```python
from build123d import *

# Parameters (mm, degrees)
SKETCH1_W               = 265
SKETCH1_H               = 340
BOSS_EXTRUDE1_DEPTH     = 50
SKETCH2_R               = 7.5
BOSS_EXTRUDE2_DEPTH     = 80
SKETCH7_R               = 7.5
BOSS_EXTRUDE3_DEPTH     = 80
SKETCH8_R               = 7.5
CUT_EXTRUDE1_DEPTH      = 410
SKETCH9_R               = 7.5
CUT_EXTRUDE2_DEPTH      = 410
CUT_EXTRUDE4_DEPTH      = 463.803826299
CUT_EXTRUDE4_DEPTH_BACK = 463.803826299


with BuildPart() as part:
    # Sketch1 → Boss-Extrude1 (new body)
    with BuildSketch(Plane.XY):
        Polygon((-7.287721529, 248.848476773), (17.712278471, 248.848476773), (17.712278471, -351.151523227), (-7.287721529, -351.151523227), (-7.287721529, -271.151523227), (-272.287721529, -271.151523227), (-272.287721529, -351.151523227), (-297.287721529, -351.151523227), (-297.287721529, 248.848476773), (-272.287721529, 248.848476773), (-272.287721529, 168.848476773), (-7.287721529, 168.848476773), align=None)
        with Locations((-139.787721529, -51.151523227)):
            Rectangle(SKETCH1_W, SKETCH1_H, mode=Mode.SUBTRACT)
    extrude(amount=BOSS_EXTRUDE1_DEPTH)

    # Sketch2 → Boss-Extrude2 (add)
    with BuildSketch(Plane(origin=(17.712278471, 0, 0), x_dir=(0, 0, -1), z_dir=(1, 0, 0))):
        with Locations((-26.558504248, -51.151523227)):
            Circle(SKETCH2_R)
    extrude(amount=-BOSS_EXTRUDE2_DEPTH)

    # Sketch7 → Boss-Extrude3 (add)
    with BuildSketch(Plane.ZY.offset(297.287721529)):
        with Locations((25, -51.151523227)):
            Circle(SKETCH7_R)
    extrude(amount=-BOSS_EXTRUDE3_DEPTH)

    # Sketch8 → Cut-Extrude1 (cut)
    with BuildSketch(Plane.ZY.offset(297.287721529)):
        with Locations((25, -331.151523227)):
            Circle(SKETCH8_R)
    extrude(amount=-CUT_EXTRUDE1_DEPTH, mode=Mode.SUBTRACT)

    # Sketch9 → Cut-Extrude2 (cut)
    with BuildSketch(Plane.ZY.offset(297.287721529)):
        with Locations((25, 228.848476773)):
            Circle(SKETCH9_R)
    extrude(amount=-CUT_EXTRUDE2_DEPTH, mode=Mode.SUBTRACT)

    # Sketch11 → Cut-Extrude4 (cut, two sides: drawn at the far end of the back side and taken through both)
    with BuildSketch(Plane(origin=(0, 0, 0), x_dir=(0, 0, -1), z_dir=(1, 0, 0)).offset(-CUT_EXTRUDE4_DEPTH_BACK)):
        Polygon((-50, -351.151523227), (-28, -351.151523227), (-50, -300.151523227), align=None)
    extrude(amount=CUT_EXTRUDE4_DEPTH + CUT_EXTRUDE4_DEPTH_BACK, mode=Mode.SUBTRACT)


solid = part.part
```
Design review of the part built by this model. Coordinates are the model's own, in mm. A direction names the side the tool comes from. Coordinates: 2 decimals unless noted, no trailing zeros. Order: outer loops, then holes, each group sorted by start corner. A loop starts at its lowest first (then second) coordinate and runs counter-clockwise, first axis right, second up. Notation, with made-up numbers: M 75.25,68.25 L 100.25,68.25 A28 ccw 100.25,101.25 Z; hole C -15,33.25 d6. An arc over 180 degrees is marked long. Answer as a JSON object with one key per item and string values. Group by question number.
1) Mouldability with a two-part tool opening along X and no side actions: class faces 1 (the flat face through (-297.288, -47, 25)), 2 (the flat face through (-278, -47, 0)), 3 (the flat face through (-142, -221.152, 25)) as pulls with the +X half, pulls with the -X half, needs draft (parallel to the pull), parting line crosses it, or undercut.
2) Add section C-C, the plane z = 11. Write out the cut boundary in (x, y).
3) Add section A-A, the plane y = 0.5. Write out the cut boundary in (x, z).
4) Add section D-D, the plane z = 39.5. Write out the cut boundary in (x, y).
5) For pin 1 (1.5 mm diameter, centred on x = -114.5, z = 7, fed in from -Y); pin 2 (2 mm diameter, centred on x = -27, z = 34, fed in from +Y); pin 3 (25 mm diameter, centred on y = -329.5, z = 18.5, fed in from -X), all flat-tipped, find the tip position at first contact; note any pin that passes through.
6) Add section B-B, the plane x = -205. Write out the cut boundary in (y, z), then the cut area to 3 significant figures.
7) Tool access review of faces 4 (the flat face through (-62.288, -51, 27)), 5 (the flat face through (-7.288, -303, 19)), 6 (the flat face through (-272.288, 209, 25)), 7 (the cylindrical face through (-245.173, -46.083, 19.472)): name each direction out of +Z, -Z, +X, -X, +Y, -Y from which nothing blocks a thin tool from reaching the whole face with its end or side.
8) Wall thickness on L1, parallel to Y at x = -26, z = 27; L2, parallel to Y at x = 12.25, z = 25; L3, parallel to X at y = -125.5, z = 38: over which ranges is each line inside the solid? List them lowest first.
Computed values:
{
 "1": {"face 1": "pulls with the -X half", "face 2": "needs draft", "face 3": "undercut"},
 "2": {"outline": "M -297.29,-351.15 L -272.29,-351.15 L -272.29,-271.15 L -7.29,-271.15 L -7.29,-351.15 L 17.71,-351.15 L 17.71,248.85 L -7.29,248.85 L -7.29,168.85 L -272.29,168.85 L -272.29,248.85 L -297.29,248.85 Z; hole M -272.29,-221.15 L -7.29,-221.15 L -7.29,118.85 L -272.29,118.85 Z"},
 "3": {"outline": "M -297.29,0 L -272.29,0 L -272.29,50 L -297.29,50 Z; M -7.29,0 L 17.71,0 L 17.71,50 L -7.29,50 Z"},
 "4": {"outline": "M -297.29,-324.49 L -272.29,-324.49 L -272.29,-271.15 L -7.29,-271.15 L -7.29,-324.49 L 17.71,-324.49 L 17.71,248.85 L -7.29,248.85 L -7.29,168.85 L -272.29,168.85 L -272.29,248.85 L -297.29,248.85 Z; hole M -272.29,-221.15 L -7.29,-221.15 L -7.29,118.85 L -272.29,118.85 Z"},
 "5": {"pin 1": "stops at y = -271.15", "pin 2": "stops at y = 168.85", "pin 3": "stops at x = -297.29"},
 "6": {"outline": "M -271.15,0 L -221.15,0 L -221.15,50 L -271.15,50 Z; M 118.85,0 L 168.85,0 L 168.85,50 L 118.85,50 Z", "area": "5,000 mm^2"},
 "7": {"face 4": "+Z, -Z", "face 5": "+Z, -Z, -Y", "face 6": "+Z, -Z, +Y", "face 7": "none"},
 "8": {"L1": "y = -271.15 to -221.15, -58.64 to -43.66, 118.85 to 168.85", "L2": "y = -351.15 to -338.65, -323.65 to 221.35, 236.35 to 248.85", "L3": "x = -297.29 to -272.29, -7.29 to 17.71"}
}
